The model under review builds one solid part; all positions refer to its coordinate system, in mm. Round coordinates to 2 decimals unless told otherwise and drop trailing zeros. Write each loop counter-clockwise with the first axis right and the second up, starting at its lowest first coordinate (ties: lowest second). Pieces come first, ordered by that corner, then holes. Notation, with made-up numbers: (83, 4.5) -> (130, 4.5) arc R13 ccw to (130, 24.5) -> close; hole circle Ø1 at (32, 3). An arc over 180 degrees is marked (long way). Use CSV: the item, a comma, the result in double quotes. Start each with the question number.
1) Mouldability with a two-part tool opening along X and no side actions: class faces 1 (the face through (-72, 11, 11.425)), 2 (the face through (-72.957, 15.073, 13.89)) as released by +X, released by -X, zero draft, split by the parting line, or undercut.
2) Take a section at A-A, the plane x = -68.5. Give the boundary of the cut face in (y, z) (3 decimals).
3) Take a section at C-C, the plane z = 14.15. Give the boundary of the cut face in (x, y), then the cut area to 3 significant figures.
4) For pin 1 Ø1.5 at (y, z) = (20, 13) entering from -X; pin 2 Ø1 at (y, z) = (10.5, 12.5) entering from -X; pin 3 Ø1.5 at (y, z) = (16.5, 13) entering from +X, all flat-tipped, find the tip position at first contact; note any pin that passes through.
5) Take a section at B-B, the plane y = 16.75. Give the boundary of the cut face in (x, z) (3 decimals).
6) Wall thickness on probe 1 along X at (y, z) = (13.25, 13.6); probe 2 along Y at (x, z) = (-67.75, 13); probe 3 along Y at (x, z) = (-67.25, 15.65): over which ranges is each line inside the solid? List them lowest first. Write a range as [from, to].
7) Take a section at D-D, the plane y = 20. Give the boundary of the cut face in (x, z) (3 decimals), then the cut area to 3 significant figures.
from build123d import *

# Parameters (mm, degrees)
SKETCH1_R           = 7.5
SKETCH1_R_2         = 3
BOSS_EXTRUDE1_DEPTH = 3.82499
SKETCH2_R           = 7.5
SKETCH2_R_2         = 3
BOSS_EXTRUDE2_DEPTH = 1.17501
CUT_EXTRUDE1_REACH  = 7
SKETCH3_R           = 3.1


with BuildPart() as part:
    # Sketch1 → Boss-Extrude1 (new body)
    with BuildSketch(Plane.XY.offset(12.6)):
        with Locations((-69.999984325, 14.142135624)):
            Circle(SKETCH1_R)
        with Locations((-69.999984325, 14.142135624)):
            Circle(SKETCH1_R_2, mode=Mode.SUBTRACT)
    extrude(amount=BOSS_EXTRUDE1_DEPTH)

    # Sketch2 → Boss-Extrude2 (add)
    with BuildSketch(Plane(origin=(0, 0, 12.6), x_dir=(-1, 0, 0), z_dir=(0, 0, -1))):
        with Locations((69.999984325, 14.142135624)):
            Circle(SKETCH2_R)
        with Locations((69.999984325, 14.142135624)):
            Circle(SKETCH2_R_2, mode=Mode.SUBTRACT)
    extrude(amount=BOSS_EXTRUDE2_DEPTH)

    # Sketch3 → Cut-Extrude1 (cut, up to next)
    with BuildSketch(Plane(origin=(0, 0, 11.424990227), x_dir=(-1, 0, 0), z_dir=(0, 0, -1)), mode=Mode.PRIVATE) as cut_extrude1_sk1:
        with Locations((69.999984325, 14.142135624)):
            Circle(SKETCH3_R)
    cut_extrude1_tool1 = extrude(cut_extrude1_sk1.sketch, amount=-CUT_EXTRUDE1_REACH, mode=Mode.PRIVATE) & part.part
    add(cut_extrude1_tool1.solids().sort_by_distance((-69.999984, 14.142136, 11.42499))[0], mode=Mode.SUBTRACT)


solid = part.part
Values found:
1,face 1,"zero draft"
1,face 2,"undercut"
2,outline,"(6.794, 11.425) -> (11.429, 11.425) -> (11.429, 16.425) -> (6.794, 16.425) -> close; (16.855, 11.425) -> (21.491, 11.425) -> (21.491, 16.425) -> (16.855, 16.425) -> close"
3,outline,"circle Ø15 at (-70, 14.14); hole circle Ø6.2 at (-70, 14.14)"
3,area,"147 mm²"
4,pin 1,"x = -75.49"
4,pin 2,"x = -76.81"
4,pin 3,"x = -62.67"
5,outline,"(-77.032, 11.425) -> (-71.676, 11.425) -> (-71.676, 16.425) -> (-77.032, 16.425) -> close; (-68.324, 11.425) -> (-62.968, 11.425) -> (-62.968, 16.425) -> (-68.324, 16.425) -> close"
6,probe 1,"[-77.45, -72.97], [-67.03, -62.55]"
6,probe 2,"[6.99, 12.01], [16.27, 21.3]"
6,probe 3,"[7.16, 12.71], [15.57, 21.12]"
7,outline,"(-74.684, 11.425) -> (-65.316, 11.425) -> (-65.316, 16.425) -> (-74.684, 16.425) -> close"
7,area,"46.8 mm²"
